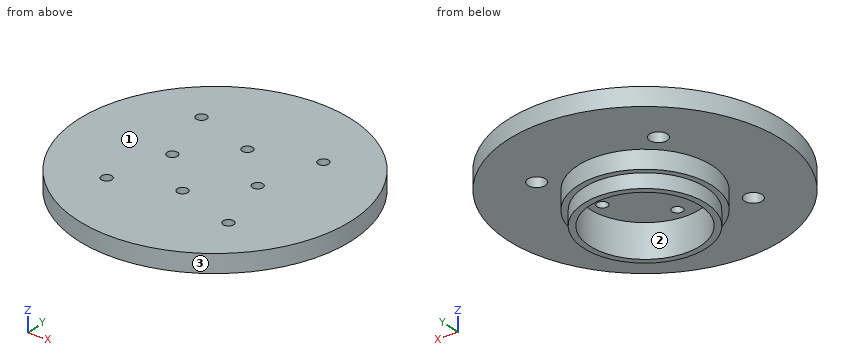
```python
from build123d import *

# Parameters (mm, degrees)
SKETCH1_R               = 45
BOSS_EXTRUDE1_DEPTH     = 6
SKETCH2_R               = 22
BOSS_EXTRUDE2_DEPTH     = 6
SKETCH3_R               = 20.1
BOSS_EXTRUDE3_DEPTH     = 4.7
SKETCH4_R               = 18.1
CUT_EXTRUDE1_DEPTH      = 11
SKETCH5_R               = 1.75
CUT_EXTRUDE2_DEPTH      = 6.7
SKETCH6_R               = 1.75
CUT_EXTRUDE3_DEPTH      = 12
CUT_EXTRUDE3_DEPTH_BACK = 6.7
SKETCH7_R               = 2.9
CUT_EXTRUDE5_DEPTH      = 3.3


with BuildPart() as part:
    # Sketch1 → Boss-Extrude1 (new body)
    with BuildSketch(Plane.XY):
        Circle(SKETCH1_R)
    extrude(amount=BOSS_EXTRUDE1_DEPTH)

    # Sketch2 → Boss-Extrude2 (add)
    with BuildSketch(Plane(origin=(0, 0, 0), x_dir=(-1, 0, 0), z_dir=(0, 0, -1))):
        Circle(SKETCH2_R)
    extrude(amount=BOSS_EXTRUDE2_DEPTH)

    # Sketch3 → Boss-Extrude3 (add)
    with BuildSketch(Plane(origin=(0, 0, -6), x_dir=(-1, 0, 0), z_dir=(0, 0, -1))):
        Circle(SKETCH3_R)
    extrude(amount=BOSS_EXTRUDE3_DEPTH)

    # Sketch4 → Cut-Extrude1 (cut)
    with BuildSketch(Plane(origin=(0, 0, -10.7), x_dir=(-1, 0, 0), z_dir=(0, 0, -1))):
        Circle(SKETCH4_R)
    extrude(amount=-CUT_EXTRUDE1_DEPTH, mode=Mode.SUBTRACT)

    # Sketch5 → Cut-Extrude2 (cut, through all)
    with BuildSketch(Plane(origin=(0, 0, 0.3), x_dir=(-1, 0, 0), z_dir=(0, 0, -1))):
        with Locations((14, 0)):
            Circle(SKETCH5_R)
        with Locations((0, -14)):
            Circle(SKETCH5_R)
        with Locations((-14, 0)):
            Circle(SKETCH5_R)
        with Locations((0, 14)):
            Circle(SKETCH5_R)
    extrude(amount=-CUT_EXTRUDE2_DEPTH, mode=Mode.SUBTRACT)

    # Sketch6 → Cut-Extrude3 (cut, two sides)
    with BuildSketch(Plane(origin=(0, 0, 0.3), x_dir=(-1, 0, 0), z_dir=(0, 0, -1))) as cut_extrude3_sk:
        with Locations((19.999991423, -20.5)):
            Circle(SKETCH6_R)
        with Locations((-19.999991423, 20.5)):
            Circle(SKETCH6_R)
        with Locations((-19.999991423, -20.5)):
            Circle(SKETCH6_R)
        with Locations((19.999991423, 20.5)):
            Circle(SKETCH6_R)
    extrude(amount=CUT_EXTRUDE3_DEPTH, mode=Mode.SUBTRACT)
    extrude(cut_extrude3_sk.sketch, amount=-CUT_EXTRUDE3_DEPTH_BACK, mode=Mode.SUBTRACT)

    # Sketch7 → Cut-Extrude5 (cut)
    with BuildSketch(Plane.XY):
        with Locations((19.999991423, 20.5)):
            Circle(SKETCH7_R)
        with Locations((-19.999991423, 20.5)):
            Circle(SKETCH7_R)
        with Locations((-19.999991423, -20.5)):
            Circle(SKETCH7_R)
        with Locations((19.999991423, -20.5)):
            Circle(SKETCH7_R)
    extrude(amount=CUT_EXTRUDE5_DEPTH, mode=Mode.SUBTRACT)


solid = part.part
```
Geometry check sheet. Reference: the model listing, model coordinates, mm. Face numbers are marked on the shaded views. Give positions to 0.01 mm unless a question says otherwise; leave off trailing zeros. Loops run counter-clockwise (first coordinate to the right, second up) from the corner with the lowest first, then second, coordinate; pieces in that order, holes last. Notation, with made-up numbers: M 46.25,-37.5 L 65.25,-37.5 A31 ccw 65.25,-0.5 Z; hole C 1,44 d9. An arc over 180 degrees is marked long. Write item = value, one per line.
(1) Gauge pin test, flat ends, axial feed: pin 1 Ø4 at (y, z) = (27.5, -3) entering from +X; pin 2 Ø4.5 at (x, y) = (-20, -20.5) entering from -Z; pin 3 Ø8 at (y, z) = (-15.5, 1.5) entering from +X; pin 4 Ø1.5 at (x, z) = (-20.5, 3.5) entering from -Y. Record the tip position at first contact, or that the pin passes through.
Answer below:
pin_1 = through
pin_2 = 3.3
pin_3 = 43.51
pin_4 = -40.43
(2) Sectioned sample at A-A, the plane z = 2. State how many separate pieces and enclosed holes the cut face has, plus the area to 3 significant figures.
Answer below:
separate_pieces = 1
enclosed_holes = 8
area = 6,220 mm2
(3) Release check for a two-part mould opening along Y. For the marked faces 1, 2 and 3 record: released by +Y, released by -Y, zero draft, split by the parting line, or undercut.
Answer below:
face_1 = zero draft
face_2 = undercut
face_3 = split by the parting line
(4) Material ranges on line 1 (Y direction, x = 0, z = 3); line 2 (Z direction, x = -7, y = 28.5); line 3 (Y direction, x = -14.5, z = -2), recorded low to high. Write a range as [from, to].
Answer below:
line_1 = [-45, -15.75], [-12.25, 12.25], [15.75, 45]
line_2 = [0, 6]
line_3 = [-16.55, -10.83], [10.83, 16.55]
(5) Sectioned sample at B-B, the plane x = 0. Record the cut outline in (y, z), plus the area to 3 significant figures.
Answer below:
outline = M -45,0 L -22,0 L -22,-6 L -20.1,-6 L -20.1,-10.7 L -18.1,-10.7 L -18.1,0.3 L -15.75,0.3 L -15.75,6 L -45,6 Z; M -12.25,0.3 L 12.25,0.3 L 12.25,6 L -12.25,6 Z; M 15.75,0.3 L 18.1,0.3 L 18.1,-10.7 L 20.1,-10.7 L 20.1,-6 L 22,-6 L 22,0 L 45,0 L 45,6 L 15.75,6 Z
area = 555 mm2
(6) Sectioned sample at D-D, the plane z = -8.5. Record the cut outline in (x, y).
Answer below:
outline = C 0,0 d40.2; hole C 0,0 d36.2
